For this review, take the finished solid that the model builds, in its own axes (mm). A direction names the side the tool comes from. Round coordinates to 2 decimals unless told otherwise and drop trailing zeros. Order: outer loops, then holes, each group sorted by start corner. A loop starts at its lowest first (then second) coordinate and runs counter-clockwise, first axis right, second up.
from build123d import *

# Parameters (mm, degrees)
F1_DEPTH       = 95.25
F2_DEPTH       = 19.05
F5_DEPTH       = 69.85
F7_D           = 6.35
F7_DEPTH       = 25.4
F7_CBORE_D     = 6.35
F7_CBORE_DEPTH = 6.35
F9_ANGLE       = 180


with BuildPart() as f1:
    # F0 (on Top) → F1 (new body)
    with BuildSketch(Plane.XY):
        with BuildLine():
            Line((-14.2875, -14.2875), (-14.2875, 23.409222))
            ThreePointArc((-14.2875, 23.409222), (-21.152732, 18.88963), (-23.8125, 11.1125))
            Line((-23.8125, 11.1125), (-23.8125, -11.1125))
            ThreePointArc((-23.8125, -11.1125), (-20.092756, -20.092756), (-11.1125, -23.8125))
            Line((-11.1125, -23.8125), (11.1125, -23.8125))
            ThreePointArc((11.1125, -23.8125), (18.88963, -21.152732), (23.409222, -14.2875))
            Line((23.409222, -14.2875), (-14.2875, -14.2875))
        make_face()
        with BuildLine():
            Line((11.1125, 23.8125), (-11.1125, 23.8125))
            ThreePointArc((-11.1125, 23.8125), (-12.712755, 23.711277), (-14.2875, 23.409222))
            Line((-14.2875, 23.409222), (-14.2875, -14.2875))
            Line((-14.2875, -14.2875), (23.409222, -14.2875))
            ThreePointArc((23.409222, -14.2875), (23.711277, -12.712755), (23.8125, -11.1125))
            Line((23.8125, -11.1125), (23.8125, 11.1125))
            ThreePointArc((23.8125, 11.1125), (20.092756, 20.092756), (11.1125, 23.8125))
        make_face()
    extrude(amount=-F1_DEPTH)

    # F0 (on Top) → F2 (cut)
    with BuildSketch(Plane.XY):
        with BuildLine():
            Line((11.1125, 23.8125), (-11.1125, 23.8125))
            ThreePointArc((-11.1125, 23.8125), (-12.712755, 23.711277), (-14.2875, 23.409222))
            Line((-14.2875, 23.409222), (-14.2875, -14.2875))
            Line((-14.2875, -14.2875), (23.409222, -14.2875))
            ThreePointArc((23.409222, -14.2875), (23.711277, -12.712755), (23.8125, -11.1125))
            Line((23.8125, -11.1125), (23.8125, 11.1125))
            ThreePointArc((23.8125, 11.1125), (20.092756, 20.092756), (11.1125, 23.8125))
        make_face()
    extrude(amount=-F2_DEPTH, mode=Mode.SUBTRACT)

    # F3 (on face) → F5 (cut, through all)
    with BuildSketch(Plane(origin=(0, 0, -95.25), x_dir=(1, 0, 0), z_dir=(0, 0, -1))):
        with BuildLine():
            Line((17.4625, -11.1125), (17.4625, 11.1125))
            ThreePointArc((17.4625, 11.1125), (15.602628, 15.602628), (11.1125, 17.4625))
            Line((11.1125, 17.4625), (-11.1125, 17.4625))
            ThreePointArc((-11.1125, 17.4625), (-15.602628, 15.602628), (-17.4625, 11.1125))
            Line((-17.4625, 11.1125), (-17.4625, -11.1125))
            ThreePointArc((-17.4625, -11.1125), (-15.602628, -15.602628), (-11.1125, -17.4625))
            Line((-11.1125, -17.4625), (11.1125, -17.4625))
            ThreePointArc((11.1125, -17.4625), (15.602628, -15.602628), (17.4625, -11.1125))
        make_face()
    extrude(amount=-F5_DEPTH, mode=Mode.SUBTRACT)

    # F7
    with Locations(Plane.XY.offset(-19.05)):
        with Locations((4.560861, 4.560861)):
            CounterBoreHole(F7_D / 2, F7_CBORE_D / 2, F7_CBORE_DEPTH, depth=F7_DEPTH)


with BuildPart() as f1_1:
    # F9: moved
    add(f1.part.rotate(Axis((0, 0, 6.654953), (0, 0, 1)), F9_ANGLE))


solid = f1_1.part
(1) Clearance check with flat-ended pins moving along their axes: P1, Ø11.5, axis at x = -5.5, y = -6, coming from the +Z side; P2, Ø12, axis at y = -18.5, z = -10.5, coming from the +X side; P3, Ø10, axis at y = 17.5, z = -9.5, coming from the -X side; P4, Ø1, axis at x = -2, y = 16, coming from the +Z side. State where each tip first meets the part, or that it passes through.
(2) Draft analysis for pull direction Y (two halves, no side actions). For faces 4 (the face through (15.553, 15.652, -60.814)), 5 (the face through (-15.652, 15.553, -60.814)), 6 (the face through (20.191, 19.993, -46.958)), 7 (the face through (-4, 14.288, -9)), state which applies: pulls with the +Y half, pulls with the -Y half, needs draft (parallel to the pull), parting line crosses it, or undercut.
(3) Wall thickness on L1, parallel to Y at x = 0.5, z = -39; L2, parallel to Z at x = -17, y = -7: over which ranges is each line inside the solid? List them lowest first.
(4) Tool access review of faces 1 (the face through (14.288, -5, -9)), 2 (the face through (-17.462, 0, -61)), 3 (the face through (-5.25, -1.46, -22.27)): name each direction out of +Z, -Z, +X, -X, +Y, -Y from which nothing blocks a thin tool from reaching the whole face with its end or side.
(5) Add section C-C on z = -70. Give the boundary of the cut face in (x, y), plus the area to 3 significant figures.
(6) Add section B-B on x = -4.5. Give the boundary of the cut face in (y, z), plus the area to 3 significant figures.
(7) Add section A-A on y = 7.5. Give the boundary of the cut face in (x, z), plus the area to 3 significant figures.
Here are the results:
1. P1: stops at z = -19.05
1. P2: stops at x = 23.74
1. P3: stops at x = -23.41
1. P4: stops at z = 0
2. face 4: undercut
2. face 5: undercut
2. face 6: pulls with the +Y half
2. face 7: pulls with the -Y half
3. L1: y = -23.81 to -17.46, 17.46 to 23.81
3. L2: z = -25.4 to -19.05
4. face 1: +Z, -X, -Y
4. face 2: -Z
4. face 3: +Z, -Z
5. outline: (-23.81, -11.11) arc R12.7 ccw to (-11.11, -23.81) - (11.11, -23.81) arc R12.7 ccw to (14.29, -23.41) arc R12.7 ccw to (23.81, -11.11) - (23.81, 11.11) arc R12.7 ccw to (11.11, 23.81) - (-11.11, 23.81) arc R12.7 ccw to (-23.41, 14.29) arc R12.7 ccw to (-23.81, 11.11) - close; hole (-17.46, -11.11) arc R6.35 ccw to (-11.11, -17.46) - (11.11, -17.46) arc R6.35 ccw to (17.46, -11.11) - (17.46, 11.11) arc R6.35 ccw to (11.11, 17.46) - (-11.11, 17.46) arc R6.35 ccw to (-17.46, 11.11) - close
5. area: 945 mm2
6. outline: (-23.81, -95.25) - (-17.46, -95.25) - (-17.46, -25.4) - (-7.74, -25.4) - (-7.74, -19.05) - (-23.81, -19.05) - close; (-1.39, -25.4) - (17.46, -25.4) - (17.46, -95.25) - (23.81, -95.25) - (23.81, 0) - (14.29, 0) - (14.29, -19.05) - (-1.39, -19.05) - close
6. area: 1,330 mm2
7. outline: (-23.81, -95.25) - (-17.46, -95.25) - (-17.46, -25.4) - (17.46, -25.4) - (17.46, -95.25) - (23.81, -95.25) - (23.81, 0) - (14.29, 0) - (14.29, -19.05) - (-23.81, -19.05) - close
7. area: 1,370 mm2
